Geometry: final body of the model. Coordinates: model frame, mm. A direction names the side the tool comes from. Round coordinates to 2 decimals unless told otherwise and drop trailing zeros. Write each loop counter-clockwise with the first axis right and the second up, starting at its lowest first coordinate (ties: lowest second). Pieces come first, ordered by that corner, then holes. Notation, with made-up numbers: M 59,85.5 L 108,85.5 A21 cw 108,114.5 Z; hole C 22,43 d7. An arc over 180 degrees is marked long. Use one line per item in the form item = value. Start each with the question number.
from build123d import *

# Parameters (mm, degrees)
SKETCH_1_R      = 20
SKETCH_1_R_2    = 17
EXTRUDE_1_DEPTH = 22
SKETCH_2_R      = 25
EXTRUDE_2_DEPTH = 10
CHAMFER_1_SIZE  = 3


with BuildPart() as part:
    # 草图1 → 凸台-拉伸1 (new body)
    with BuildSketch(Plane.XY):
        Circle(SKETCH_1_R)
        Circle(SKETCH_1_R_2, mode=Mode.SUBTRACT)
    extrude(amount=EXTRUDE_1_DEPTH)

    # 草图2 → 凸台-拉伸2 (add)
    with BuildSketch(Plane(origin=(0, 0, 0), x_dir=(-1, 0, 0), z_dir=(0, 0, -1))):
        Circle(SKETCH_2_R)
    extrude(amount=EXTRUDE_2_DEPTH)

    # 倒角1
    chamfer_1_edges = [part.edges().sort_by_distance(p)[0] for p in [
        (25, 0, 0),
        (25, 0, -10),
    ]]
    chamfer(chamfer_1_edges, length=CHAMFER_1_SIZE)


solid = part.part
1. Section query A-A (y = 0). Return loops of the section in (x, z).
2. Contact query for flat-ended pins moving along their axis: pin 1 (1.5 mm diameter, centred on x = 17, z = 9.5, fed in from -Y); pin 2 (12 mm diameter, centred on x = -19.5, y = -19.5, fed in from -Z); pin 3 (2 mm diameter, centred on x = 8.5, z = 17.5, fed in from +Y); pin 4 (5 mm diameter, centred on x = 14, z = 5.5, fed in from +Y). Output: stop coordinate, or through.
3. Section query C-C (z = 6.5). Return loops of the section in (x, y).
4. Ray query, probe 1 along Y at (x, z) = (0, 5); probe 2 along Z at (x, y) = (-4.5, -11.5); probe 3 along X at (y, z) = (-2.5, 17). Return the intervals inside material, ascending.
5. Set-up query: faces 4 (the face through (0, 0, -10)), 5 (the face through (-4.336, -19.524, 10.846)). Return all of +Z, -Z, +X, -X, +Y, -Y with unobstructed straight access to the full face (end or side cutting, diameter ignored); none if empty.
6. Pull-direction query (X, two-part tool) for faces 1 (the face through (-23.846, 7.509, -4.972)), 2 (the face through (9.139, 14.334, 10.846)), 3 (the face through (-9, -15, 22)); classes: released by +X, released by -X, zero draft, split by the parting line, or undercut.
Checks:
q1.outline = M -25,-7 L -22,-10 L 22,-10 L 25,-7 L 25,-3 L 22,0 L 20,0 L 20,22 L 17,22 L 17,0 L -17,0 L -17,22 L -20,22 L -20,0 L -22,0 L -25,-3 Z
q2.pin_1 = -11.66
q2.pin_2 = -10
q2.pin_3 = 18.54
q2.pin_4 = 16.36
q3.outline = C 0,0 d40; hole C 0,0 d34
q4.probe_1 = -20 to -17, 17 to 20
q4.probe_2 = -10 to 0
q4.probe_3 = -19.84 to -16.82, 16.82 to 19.84
q5.face_4 = -Z, +X, -X, +Y, -Y
q5.face_5 = +Z
q6.face_1 = split by the parting line
q6.face_2 = undercut
q6.face_3 = zero draft
